The model under review builds one solid part; all positions refer to its coordinate system, in mm. Give positions to 0.01 mm unless a question says otherwise; leave off trailing zeros. Order: outer loops, then holes, each group sorted by start corner. A loop starts at its lowest first (then second) coordinate and runs counter-clockwise, first axis right, second up. Notation, with made-up numbers: (-3, 72.25) - (2, 72.25) arc R23 ccw to (2, 105.25) - close; hole circle Ø3 at (32.25, 78). An arc over 180 degrees is marked (long way). Use CSV: the item, a comma, the result in double quotes. Start each with the question number.
1. To check wall thickness, follow line 1 (X direction, y = 15.5, z = 1.5) (3 decimals); line 2 (Y direction, x = -19, z = 2.45); line 3 (Y direction, x = -15.5, z = 3.05). State the ranges of each line that lie inside material, in increasing order. Write a range as [from, to].
2. Take a section at B-B, the plane x = -23.5. State the section outline as (y, z) points (3 decimals).
3. Take a section at A-A, the plane y = 15.5. State the section outline as (x, z) points (3 decimals), then the cut area to 3 significant figures.
4. Take a section at C-C, the plane y = 27. Count the separate pieces of the cut face and the enclosed holes in it, then the cut area to 3 significant figures.
```python
from build123d import *

# Parameters (mm, degrees)
F0_W     = 142.875
F0_H     = 50.8
F0_R     = 11.1125
F1_DEPTH = 3.175
F2_W     = 3.175
F2_H     = 6.35
F3_DEPTH = 3.175


with BuildPart() as f1:
    # F0 (on Top) → F1 (new body)
    with BuildSketch(Plane.XY):
        with Locations((-71.4375, 25.4)):
            Rectangle(F0_W, F0_H)
        with Locations((-122.2375, 36.5125)):
            Circle(F0_R, mode=Mode.SUBTRACT)
        with Locations((-20.6375, 36.5125)):
            Circle(F0_R, mode=Mode.SUBTRACT)
    extrude(amount=F1_DEPTH)

    # F2 (on face) → F3 (cut, through all)
    with BuildSketch(Plane.XY.offset(3.175)):
        with Locations((-4.7625, 41.275)):
            Rectangle(F2_W, F2_H)
        with Locations((-4.7625, 28.575)):
            Rectangle(F2_W, F2_H)
        with Locations((-4.7625, 15.875)):
            Rectangle(F2_W, F2_H)
        with Locations((-138.1125, 41.275)):
            Rectangle(F2_W, F2_H)
        with Locations((-138.1125, 28.575)):
            Rectangle(F2_W, F2_H)
        with Locations((-138.1125, 15.875)):
            Rectangle(F2_W, F2_H)
        with Locations((-73.025, 41.275)):
            Rectangle(F2_W, F2_H)
        with Locations((-73.025, 28.575)):
            Rectangle(F2_W, F2_H)
    extrude(amount=-F3_DEPTH, mode=Mode.SUBTRACT)


solid = f1.part
```
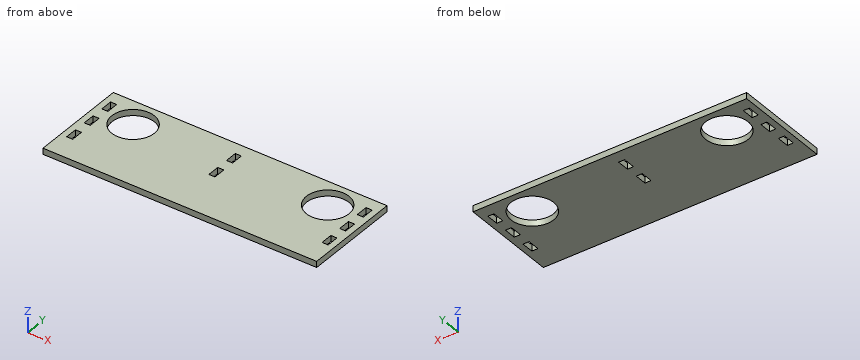
Determined:
1,line 1,"x = [-142.875, -139.7], [-136.525, -6.35], [-3.175, 0]"
1,line 2,"y = [0, 25.52], [47.5, 50.8]"
1,line 3,"y = [0, 26.66], [46.37, 50.8]"
2,outline,"(0, 0) - (25.775, 0) - (25.775, 3.175) - (0, 3.175) - close; (47.25, 0) - (50.8, 0) - (50.8, 3.175) - (47.25, 3.175) - close"
3,outline,"(-142.875, 0) - (-139.7, 0) - (-139.7, 3.175) - (-142.875, 3.175) - close; (-136.525, 0) - (-6.35, 0) - (-6.35, 3.175) - (-136.525, 3.175) - close; (-3.175, 0) - (0, 0) - (0, 3.175) - (-3.175, 3.175) - close"
3,area,"433 mm²"
4,separate pieces,"6"
4,enclosed holes,"0"
4,area,"350 mm²"
